```python
from build123d import *

# Parameters (mm, degrees)
SKETCH2_W           = 90
SKETCH2_H           = 54
SKETCH2_R           = 1.5
BOSS_EXTRUDE1_DEPTH = 2
SKETCH2_4_W         = 2
SKETCH2_4_H         = 2
BOSS_EXTRUDE3_DEPTH = 4


with BuildPart() as part:
    # Sketch2 → Boss-Extrude1 (new body)
    with BuildSketch(Plane(origin=(0, 1, 0), x_dir=(1, 0, 0), z_dir=(0, 1, 0))):
        Rectangle(SKETCH2_W, SKETCH2_H)
        with Locations(Location((-27.8, 9.7, 0), (0, 0, 270))):
            Circle(SKETCH2_R, mode=Mode.SUBTRACT)
        with Locations(Location((-27.8, -9.7, 0), (0, 0, 270))):
            Circle(SKETCH2_R, mode=Mode.SUBTRACT)
        with Locations(Location((27.8, -9.7, 0), (0, 0, 270))):
            Circle(SKETCH2_R, mode=Mode.SUBTRACT)
        with Locations(Location((27.8, 9.7, 0), (0, 0, 270))):
            Circle(SKETCH2_R, mode=Mode.SUBTRACT)
    extrude(amount=BOSS_EXTRUDE1_DEPTH)

    # Sketch2_4 → Boss-Extrude3 (add)
    with BuildSketch(Plane(origin=(0, 1, 0), x_dir=(1, 0, 0), z_dir=(0, 1, 0))):
        with Locations((-41, 23)):
            Rectangle(SKETCH2_4_W, SKETCH2_4_H)
        with Locations((41, -23)):
            Rectangle(SKETCH2_4_W, SKETCH2_4_H)
    extrude(amount=BOSS_EXTRUDE3_DEPTH)


solid = part.part
```
Input: part model. Units: mm. Frame: model coordinates. A direction names the side the tool comes from. Give positions to 0.01 mm unless a question says otherwise; leave off trailing zeros. Order: outer loops, then holes, each group sorted by start corner. A loop starts at its lowest first (then second) coordinate and runs counter-clockwise, first axis right, second up. Notation, with made-up numbers: (48, -40) - (71, -40) arc R21 ccw to (71, -12) - close; hole circle Ø8 at (20.5, -40). An arc over 180 degrees is marked (long way). Put each result on its own line as item: value.
Item 1: Draft query along X for faces 5 (the flat face through (-42, 4, -23)), 6 (the cylindrical face through (29.065, 1.986, -8.894)), 7 (the cylindrical face through (29.065, 1.986, 10.506)), 8 (the flat face through (42, 4, 23)). Return one class per face: +X half, -X half, draft (parallel to the pull), parting line (faces both ways), or undercut.
Found:
face 5: -X half
face 6: undercut
face 7: undercut
face 8: +X half
Item 2: Section query A-A, the plane z = 9.7. Return loops of the section in (x, y).
Found:
outline: (-45, 1) - (-29.3, 1) - (-29.3, 3) - (-45, 3) - close; (-26.3, 1) - (26.3, 1) - (26.3, 3) - (-26.3, 3) - close; (29.3, 1) - (45, 1) - (45, 3) - (29.3, 3) - close
Item 3: Access query for faces 1 (the flat face through (-41, 4, -22)), 2 (the flat face through (-40, 4, -23)), 3 (the flat face through (40, 4, 23)), 4 (the flat face through (-41, 4, -24)). Directions: +Z, -Z, +X, -X, +Y, -Y. A direction counts if a zero-diameter tool reaches every point of the face in a straight line with its end or side. Return the directions, or none.
Found:
face 1: +Z, +X, -X, +Y
face 2: +Z, -Z, +X, +Y
face 3: +Z, -Z, -X, +Y
face 4: -Z, +X, -X, +Y
Item 4: Section query B-B, the plane x = 27.8. Return loops of the section in (y, z), then the cut area to 3 significant figures.
Found:
outline: (1, -27) - (3, -27) - (3, -11.2) - (1, -11.2) - close; (1, -8.2) - (3, -8.2) - (3, 8.2) - (1, 8.2) - close; (1, 11.2) - (3, 11.2) - (3, 27) - (1, 27) - close
area: 96.0 mm^2
Item 5: Ray query, L1, parallel to X at y = 2.3, z = 9.7; L2, parallel to Y at x = 8, z = -2.5. Return the intervals inside material, ascending. Write a range as from..to.
Found:
L1: x = -45..-29.3, -26.3..26.3, 29.3..45
L2: y = 1..3
Item 6: Contact query for flat-ended pins moving along their axis: pin 1 (16 mm diameter, centred on x = 6.5, z = 8, fed in from +Y); pin 2 (2 mm diameter, centred on y = 4.5, z = 23, fed in from -X); pin 3 (0.6 mm diameter, centred on x = -41.5, y = 4.5, fed in from -Z). Output: stop coordinate, or through.
Found:
pin 1: stops at y = 3
pin 2: stops at x = 40
pin 3: stops at z = -24
Item 7: Section query D-D, the plane z = 23. Return loops of the section in (x, y).
Found:
outline: (-45, 1) - (45, 1) - (45, 3) - (42, 3) - (42, 5) - (40, 5) - (40, 3) - (-45, 3) - close
Item 8: Section query C-C, the plane y = 4.1. Return loops of the section in (x, z).
Found:
outline: (-42, -24) - (-40, -24) - (-40, -22) - (-42, -22) - close; (40, 22) - (42, 22) - (42, 24) - (40, 24) - close
